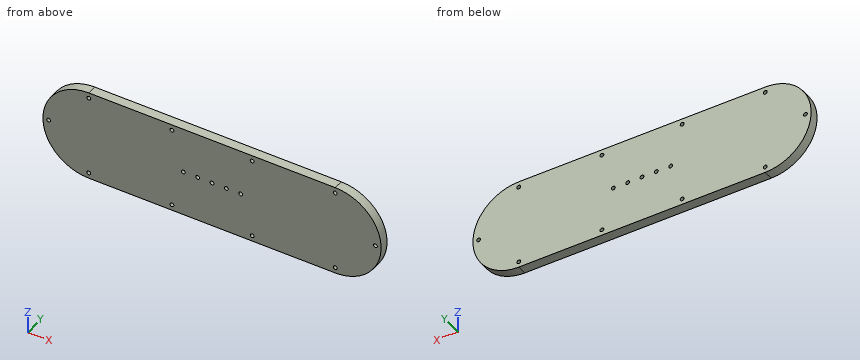
```python
from build123d import *

# Parameters (mm, degrees)
F0_R     = 2
F1_DEPTH = 10


with BuildPart() as f1:
    # F0 (on Front) → F1 (new body)
    with BuildSketch(Plane.XZ):
        with BuildLine():
            ThreePointArc((129, -48), (177, 0), (129, 48))
            Line((129, 48), (0, 48))
            Line((0, 48), (-129, 48))
            ThreePointArc((-129, 48), (-177, 0), (-129, -48))
            Line((-129, -48), (0, -48))
            Line((0, -48), (129, -48))
        make_face()
        with Locations((-129, -42)):
            Circle(F0_R, mode=Mode.SUBTRACT)
        with Locations((-42, -42)):
            Circle(F0_R, mode=Mode.SUBTRACT)
        with Locations((42, -42)):
            Circle(F0_R, mode=Mode.SUBTRACT)
        with Locations((129, -42)):
            Circle(F0_R, mode=Mode.SUBTRACT)
        with Locations((-171, 0)):
            Circle(F0_R, mode=Mode.SUBTRACT)
        with Locations((-30, 0)):
            Circle(F0_R, mode=Mode.SUBTRACT)
        with Locations((-15, 0)):
            Circle(F0_R, mode=Mode.SUBTRACT)
        with Locations((-129, 42)):
            Circle(F0_R, mode=Mode.SUBTRACT)
        with Locations((-42, 42)):
            Circle(F0_R, mode=Mode.SUBTRACT)
        Circle(F0_R, mode=Mode.SUBTRACT)
        with Locations((15, 0)):
            Circle(F0_R, mode=Mode.SUBTRACT)
        with Locations((30, 0)):
            Circle(F0_R, mode=Mode.SUBTRACT)
        with Locations((171, 0)):
            Circle(F0_R, mode=Mode.SUBTRACT)
        with Locations((42, 42)):
            Circle(F0_R, mode=Mode.SUBTRACT)
        with Locations((129, 42)):
            Circle(F0_R, mode=Mode.SUBTRACT)
    extrude(amount=F1_DEPTH)


solid = f1.part
```
Could you check a few things on this model? Use its own coordinates, in mm. Round coordinates to 2 decimals unless told otherwise and drop trailing zeros. Loops run counter-clockwise (first coordinate to the right, second up) from the corner with the lowest first, then second, coordinate; pieces in that order, holes last.
Q1. I want a section at B-B (z = 22.5). Write out the boundary of the cut face in (x, y).
Q2. For P1, Ø4, axis at y = -4.5, z = -26, coming from the +X side, with a flat end and sliding along its axis, tell me the tip position at first contact or that it passes through.
Q3. Please list where these lines run through material, in increasing order: L1, parallel to Z at x = -42, y = -4; L2, parallel to Z at x = -30, y = -2.5; L3, parallel to Z at x = 130, y = -6.5.
Q4. I want a section at A-A (y = -5.25). Give the number of separate pieces and of enclosed holes in the cut face, and give its area (3 significant figures).
Answer below:
1. outline: (-171.4, -10) - (171.4, -10) - (171.4, 0) - (-171.4, 0) - close
2. P1: stops at x = 170.57
3. L1: z = -48 to -44, -40 to 40, 44 to 48
3. L2: z = -48 to -2, 2 to 48
3. L3: z = -47.99 to -43.73, -40.27 to 40.27, 43.73 to 47.99
4. separate pieces: 1
4. enclosed holes: 15
4. area: 31,800 mm2
